Geometry: see drawing. Coordinates: mm, zero at the bounding-box minimum. Give positions to 0.01 mm unless a question says otherwise; leave off trailing zeros. Loops run counter-clockwise (first coordinate to the right, second up) from the corner with the lowest first, then second, coordinate; pieces in that order, holes last. Notation, with made-up numbers: M 78,17.25 L 125,17.25 A28 cw 125,38.25 Z; hole C 38,-1 d7. An arc over 180 degrees is marked long. Use CSV: the item, a comma, the result in double quotes. Start each with the question number.
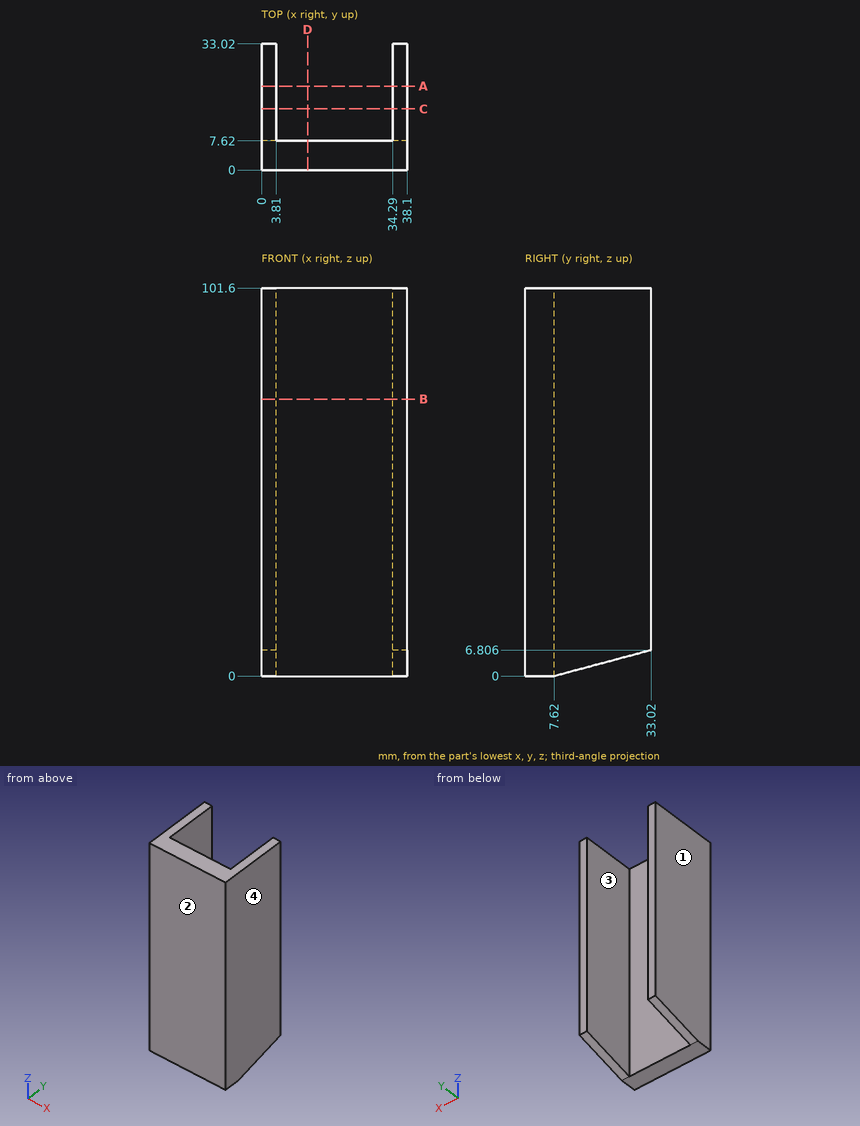
Item 1: Section B-B (z = 72.5). Output: boundary loops of the cut face in (x, y).
Item 2: First-contact query: pin 1 Ø1.5 at (x, z) = (19, 67.5) entering from +Y; pin 2 Ø8 at (x, y) = (23, 15) entering from +Z. Flat tips, straight axial feed; report the tip coordinate or a pass-through.
Item 3: Section A-A (y = 22). Output: boundary loops of the cut face in (x, z), then the cut area to 3 significant figures.
Item 4: Section C-C (y = 16). Output: boundary loops of the cut face in (x, z), then the cut area to 3 significant figures.
Item 5: Material intervals for line 1 (X direction, y = 26.5, z = 93); line 2 (Y direction, x = 15, z = 82); line 3 (Z direction, x = 3, y = 21.5), sorted ascending.
Item 6: Section D-D (x = 12). Output: boundary loops of the cut face in (y, z).
Item 7: Mould query, pull axis X, two halves, no side actions, for the marked faces 1, 2, 3 and 4. Classes: +X half, -X half, draft (parallel to the pull), parting line (faces both ways), or undercut.
Recorded:
1,outline,"M 0,0 L 38.1,0 L 38.1,33.02 L 34.29,33.02 L 34.29,7.62 L 3.81,7.62 L 3.81,33.02 L 0,33.02 Z"
2,pin 1,"y = 7.62"
2,pin 2,"through"
3,outline,"M 0,3.85 L 3.81,3.85 L 3.81,101.6 L 0,101.6 Z; M 34.29,3.85 L 38.1,3.85 L 38.1,101.6 L 34.29,101.6 Z"
3,area,"745 mm²"
4,outline,"M 0,2.25 L 3.81,2.25 L 3.81,101.6 L 0,101.6 Z; M 34.29,2.25 L 38.1,2.25 L 38.1,101.6 L 34.29,101.6 Z"
4,area,"757 mm²"
5,line 1,"0 to 3.81, 34.29 to 38.1"
5,line 2,"0 to 7.62"
5,line 3,"3.72 to 101.6"
6,outline,"M 0,0 L 7.62,0 L 7.62,101.6 L 0,101.6 Z"
7,face 1,"-X half"
7,face 2,"draft"
7,face 3,"undercut"
7,face 4,"+X half"
